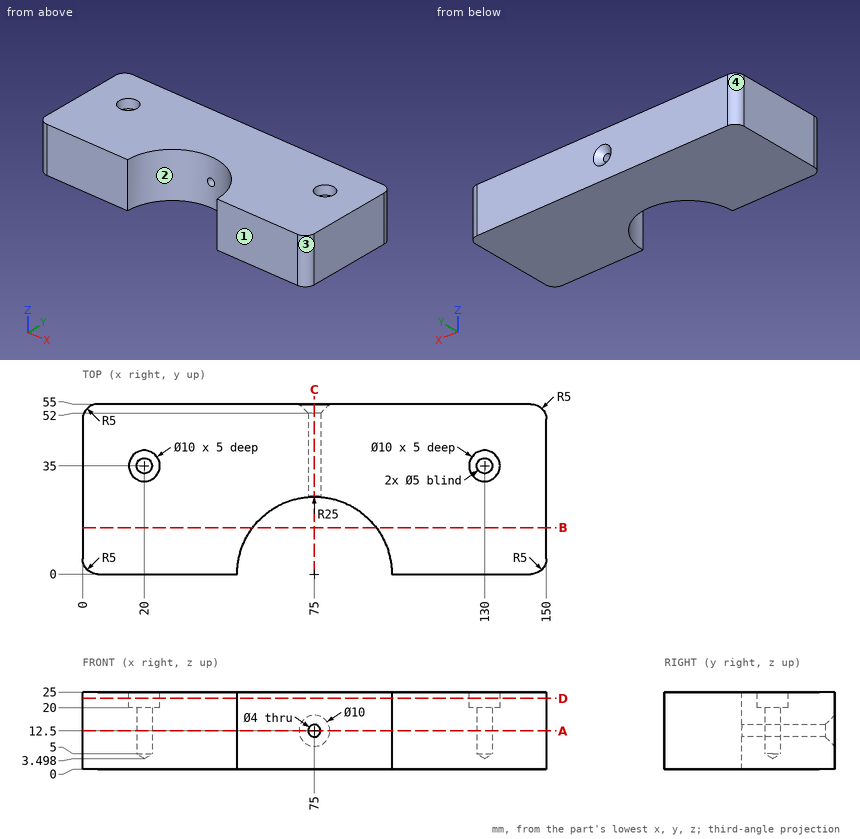
Answer from the drawing. Dimensions are ordinates in mm from the lowest x, y and z of the part. Coordinates: 2 decimals unless noted, no trailing zeros. Write each loop counter-clockwise with the first axis right and the second up, starting at its lowest first coordinate (ties: lowest second). Pieces come first, ordered by that corner, then holes. Notation, with made-up numbers: M 46,82.25 L 83,82.25 A25 ccw 83,102.25 Z; hole C -34.5,30.5 d1. An arc over 180 degrees is marked long. Use one line per item in the form item = value. Start each with the question number.
1. The mould has two halves that part along X. Classify the marked faces 1, 2, 3 and 4: released by +X, released by -X, zero draft, split by the parting line, or undercut.
2. The part is cut by section B-B (y = 15). Give the vertices of the cut face in (x, z).
3. The part is cut by section D-D (z = 23). Give the vertices of the cut face in (x, y), plus the area to 3 significant figures.
4. The part is cut by section C-C (x = 75). Give the vertices of the cut face in (y, z).
5. Straight lines are drawn through the part: probe 1 along Y at (x, z) = (20, 21.9); probe 2 along Z at (x, y) = (75, 30.75); probe 3 along Y at (x, z) = (20, 8.25). For each, find the intervals that lie inside material, in ascending order. Write a range as from..to.
6. Each of these flat-tipped pins is pushed along its axis until it touches: P1, Ø6, axis at x = 130, y = 35, coming from the +Z side; P2, Ø6, axis at x = 58, z = 16.5, coming from the -Y side. Where does it stop, or does it pass through?
7. The part is cut by section A-A (z = 12.5). Give the vertices of the cut face in (x, y).
Evaluation:
q1.face_1 = zero draft
q1.face_2 = undercut
q1.face_3 = released by +X
q1.face_4 = released by -X
q2.outline = M 0,0 L 55,0 L 55,25 L 0,25 Z; M 95,0 L 150,0 L 150,25 L 95,25 Z
q3.outline = M 0,5 A5 ccw 5,0 L 50,0 A25 cw 100,0 L 145,0 A5 ccw 150,5 L 150,50 A5 ccw 145,55 L 5,55 A5 ccw 0,50 Z; hole C 20,35 d10; hole C 130,35 d10
q3.area = 7,090 mm^2
q4.outline = M 25,0 L 55,0 L 55,7.5 L 52,10.5 L 25,10.5 Z; M 25,14.5 L 52,14.5 L 55,17.5 L 55,25 L 25,25 Z
q5.probe_1 = 0..30, 40..55
q5.probe_2 = 0..10.5, 14.5..25
q5.probe_3 = 0..32.5, 37.5..55
q6.P1 = 20
q6.P2 = 15
q7.outline = M 0,5 A5 ccw 5,0 L 50,0 A25 cw 73,24.92 L 73,52 L 70,55 L 5,55 A5 ccw 0,50 Z; M 77,24.92 A25 cw 100,0 L 145,0 A5 ccw 150,5 L 150,50 A5 ccw 145,55 L 80,55 L 77,52 Z; hole C 20,35 d5; hole C 130,35 d5
